from build123d import *

# Parameters (mm, degrees)
F0_W     = 81
F0_H     = 9.175
F0_R     = 1.5
F1_DEPTH = 3.175


# Not quite as in the source:
# - a length typed as a fraction of an inch, garbled in the dataset ("3 / 203.2 mm" for 3/8 in), is restored


with BuildPart() as f1:
    # F0 (on Top) → F1 (new body)
    with BuildSketch(Plane.XY):
        with Locations((35.4220271409, 16.632870598)):
            Rectangle(F0_W, F0_H)
        with Locations((-0.5779728591, 16.632870598)):
            Circle(F0_R, mode=Mode.SUBTRACT)
        Polygon((3.9220271409, 15.045370598), (3.9220271409, 18.220370598), (35.4220271409, 18.220370598), (66.9220271409, 18.220370598), (66.9220271409, 15.045370598), align=None, mode=Mode.SUBTRACT)
        with Locations((71.4220271409, 16.632870598)):
            Circle(F0_R, mode=Mode.SUBTRACT)
    extrude(amount=F1_DEPTH)


solid = f1.part
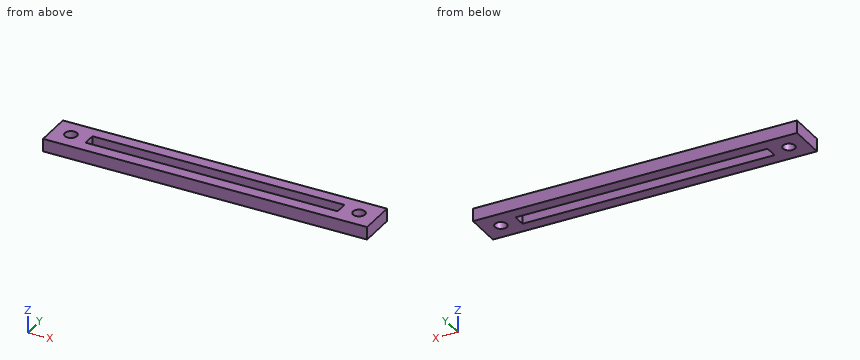
Input: part model. Units: mm. Frame: model coordinates. Round coordinates to 2 decimals unless told otherwise and drop trailing zeros. Order: outer loops, then holes, each group sorted by start corner. A loop starts at its lowest first (then second) coordinate and runs counter-clockwise, first axis right, second up. Notation, with made-up numbers: (37.5, -1) - (52.5, -1) arc R14 ccw to (52.5, 18) - close; hole circle Ø11 at (8, 5.5). An arc over 180 degrees is marked (long way). Answer as a JSON object with one key per item and string values. Group by question number.
(1) Cut plane B-B (z = 2.1). Return loops of the section in (x, y), then the cut area to 3 significant figures.
(2) Cut plane A-A (x = 55.5). Return loops of the section in (y, z) (3 decimals), then the cut area to 4 significant figures.
(3) Pin query (flat end, axial travel): P1, Ø1.8, axis at x = 71.42, y = 16.63, coming from the +Z side. Return the tip coordinate at first contact, or that it passes through.
(4) Material intervals for probe 1 along Y at (x, z) = (29, 2.05); probe 2 along X at (y, z) = (17, 0.5); probe 3 along X at (y, z) = (17.25, 2.6), sorted ascending. Write a range as from..to.
Here are the results:
{
 "1": {"outline": "(-5.08, 12.05) - (75.92, 12.05) - (75.92, 21.22) - (-5.08, 21.22) - close; hole circle Ø3 at (-0.58, 16.63); hole (3.92, 15.05) - (66.92, 15.05) - (66.92, 18.22) - (3.92, 18.22) - close; hole circle Ø3 at (71.42, 16.63)", "area": "529 mm^2"},
 "2": {"outline": "(12.045, 0) - (15.045, 0) - (15.045, 3.175) - (12.045, 3.175) - close; (18.22, 0) - (21.22, 0) - (21.22, 3.175) - (18.22, 3.175) - close", "area": "19.05 mm^2"},
 "3": {"P1": "passes through"},
 "4": {"probe 1": "y = 12.05..15.05, 18.22..21.22", "probe 2": "x = -5.08..-2.03, 0.88..3.92, 66.92..69.97, 72.88..75.92", "probe 3": "x = -5.08..-1.95, 0.79..3.92, 66.92..70.05, 72.79..75.92"}
}
